from build123d import *

# Parameters (mm, degrees)
SKETCH002_R  = 35.5
PAD001_DEPTH = 10.477
FILLET_R     = 1.57
FILLET001_R  = 1.57
SKETCH003_R  = 8


with BuildPart() as part:
    # Sketch002 → Pad001 (new body, symmetric)
    with BuildSketch(Plane.XZ):
        Circle(SKETCH002_R)
        with BuildLine():
            ThreePointArc((-2.5, 5.454356), (0, -6), (2.5, 5.454356))
            Line((2.5, 7.454356), (2.5, 5.454356))
            Line((-2.5, 7.454356), (2.5, 7.454356))
            Line((-2.5, 5.454356), (-2.5, 7.454356))
        make_face(mode=Mode.SUBTRACT)
    extrude(amount=PAD001_DEPTH, both=True)

    # Fillet
    fillet_edges = [part.edges().sort_by_distance(p)[0] for p in [
        (-35.5, 10.477, 0),
    ]]
    fillet(fillet_edges, radius=FILLET_R)

    # Fillet001
    fillet001_edges = [part.edges().sort_by_distance(p)[0] for p in [
        (-35.5, -10.477, 0),
    ]]
    fillet(fillet001_edges, radius=FILLET001_R)

    # Sketch003 → Groove (revolve, cut)
    with BuildSketch(Plane.XY):
        with Locations((42, 0)):
            Circle(SKETCH003_R)
    revolve(axis=Axis((0, 0, 0), (0, 1, 0)), mode=Mode.SUBTRACT)


solid = part.part
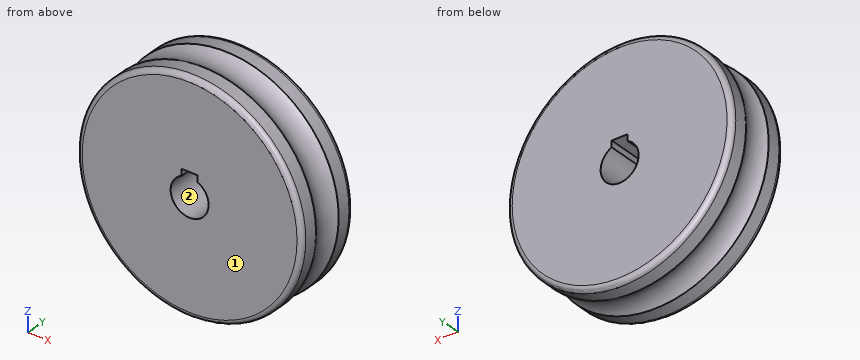
Design review of the part built by this model. Coordinates are the model's own, in mm. Face numbers are marked on the shaded views. Coordinates: 2 decimals unless noted, no trailing zeros. Order: outer loops, then holes, each group sorted by start corner. A loop starts at its lowest first (then second) coordinate and runs counter-clockwise, first axis right, second up.
Item 1: For pin 1 Ø4 at (y, z) = (5, 21.5) entering from +X; pin 2 Ø12 at (x, y) = (-17.5, -2.5) entering from +Z; pin 3 Ø1.6 at (y, z) = (-1.5, 6) entering from -X, all flat-tipped, find the tip position at first contact; note any pin that passes through.
Item 2: The part is to be moulded in two halves that separate along X. For the marked faces 1 and 2, say which applies: pulls with the +X half, pulls with the -X half, needs draft (parallel to the pull), parting line crosses it, or undercut.
Item 3: For line 1 (X direction, y = -4.75, z = 0); line 2 (Z direction, x = 0, y = 0.5); line 3 (X direction, y = -4.25, z = 0), list the stretches that pass through material, from the lowest coordinate up.
Item 4: Take a section at B-B, the plane x = 0. Write out the cut boundary in (y, z).
Item 5: Take a section at D-D, the plane y = -2.75. Write out the cut boundary in (x, z), then the cut area to 3 significant figures.
Item 6: Take a section at C-C, the plane y = -7. Write out the cut boundary in (x, z).
Item 7: Take a section at A-A, the plane z = 0. Write out the cut boundary in (x, y).
The answers:
1. pin 1: stops at x = 29.66
1. pin 2: stops at z = 33.44
1. pin 3: stops at x = -33.85
2. face 1: needs draft
2. face 2: undercut
3. line 1: x = -35.5 to -6, 6 to 35.5
3. line 2: z = -34.02 to -6, 7.45 to 34.02
3. line 3: x = -35.22 to -6, 6 to 35.22
4. outline: (-10.48, -33.93) arc R1.57 ccw to (-8.91, -35.5) - (-4.66, -35.5) arc R8 cw to (4.66, -35.5) - (8.91, -35.5) arc R1.57 ccw to (10.48, -33.93) - (10.48, -6) - (-10.48, -6) - close; (-10.48, 7.45) - (10.48, 7.45) - (10.48, 33.93) arc R1.57 ccw to (8.91, 35.5) - (4.66, 35.5) arc R8 cw to (-4.66, 35.5) - (-8.91, 35.5) arc R1.57 ccw to (-10.48, 33.93) - close
5. outline: circle Ø68.98 at (0, 0); hole (-2.5, 5.45) arc R6 ccw (long way) to (2.5, 5.45) - (2.5, 7.45) - (-2.5, 7.45) - close
5. area: 3,620 mm2
6. outline: circle Ø71 at (0, 0); hole (-2.5, 5.45) arc R6 ccw (long way) to (2.5, 5.45) - (2.5, 7.45) - (-2.5, 7.45) - close
7. outline: (-35.5, -8.91) arc R1.57 ccw to (-33.93, -10.48) - (-6, -10.48) - (-6, 10.48) - (-33.93, 10.48) arc R1.57 ccw to (-35.5, 8.91) - (-35.5, 4.66) arc R8 cw to (-35.5, -4.66) - close; (6, -10.48) - (33.93, -10.48) arc R1.57 ccw to (35.5, -8.91) - (35.5, -4.66) arc R8 cw to (35.5, 4.66) - (35.5, 8.91) arc R1.57 ccw to (33.93, 10.48) - (6, 10.48) - close
